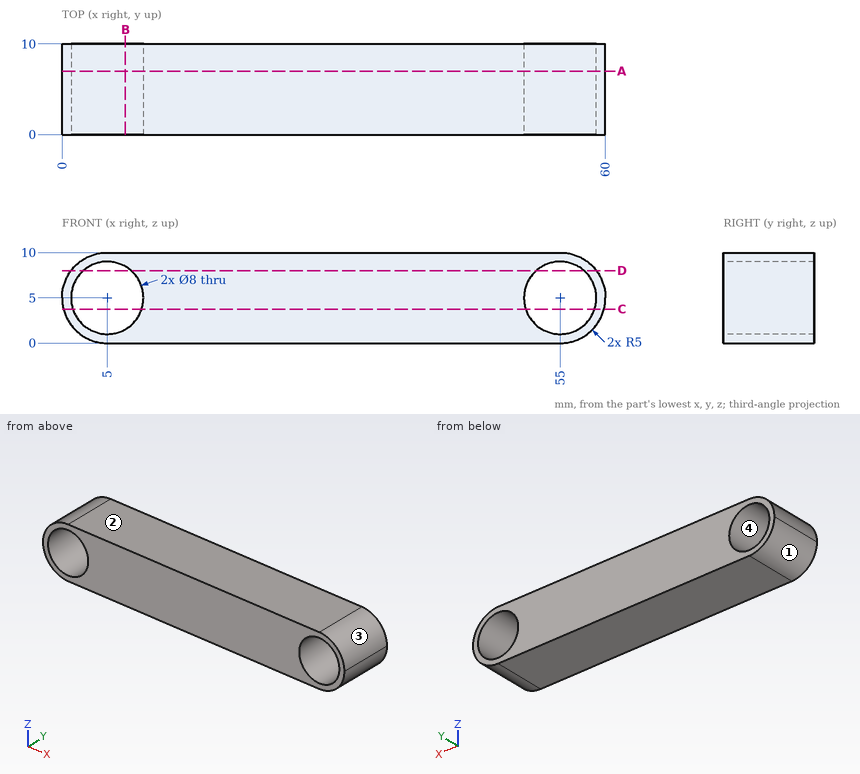
Here's the drawing with two shaded views (mm, measured from the low corner). I have some questions. Coordinates: 2 decimals unless noted, no trailing zeros. Write each loop counter-clockwise with the first axis right and the second up, starting at its lowest first coordinate (ties: lowest second). Pieces come first, ordered by that corner, then holes.
Item 1: I want a section at D-D on z = 8. Write out the boundary of the cut face in (x, y).
Item 2: I want a section at B-B on x = 7. Write out the boundary of the cut face in (y, z).
Item 3: I want a section at A-A on y = 7. Count the separate pieces of the cut face and the enclosed holes in it, and give its area (3 significant figures).
Item 4: I want a section at C-C on z = 3.75. Write out the boundary of the cut face in (x, y).
Item 5: If I drill on line 1 (X direction, y = 1.5, z = 4.75); line 2 (Z direction, x = 5, y = 8); line 3 (X direction, y = 9.25, z = 2), over which ranges is the centre line in solid material (lowest first)?
Item 6: If we mould it in two halves opening along X, with no side actions, what happens to the marked faces 1, 2, 3 and 4? For each: +X half, -X half, draft (parallel to the pull), parting line (faces both ways), or undercut.
Item 7: Will this pin go through, and if not, where does the flat tip stop? pin 1 (1.5 mm diameter, centred on y = 2, z = 3.5, fed in from +X).
Findings below:
1. outline: (1, 0) - (2.35, 0) - (2.35, 10) - (1, 10) - close; (7.65, 0) - (52.35, 0) - (52.35, 10) - (7.65, 10) - close; (57.65, 0) - (59, 0) - (59, 10) - (57.65, 10) - close
2. outline: (0, 0) - (10, 0) - (10, 1.54) - (0, 1.54) - close; (0, 8.46) - (10, 8.46) - (10, 10) - (0, 10) - close
3. separate pieces: 1
3. enclosed holes: 2
3. area: 478 mm2
4. outline: (0.16, 0) - (1.2, 0) - (1.2, 10) - (0.16, 10) - close; (8.8, 0) - (51.2, 0) - (51.2, 10) - (8.8, 10) - close; (58.8, 0) - (59.84, 0) - (59.84, 10) - (58.8, 10) - close
5. line 1: x = 0.01 to 1.01, 8.99 to 51.01, 58.99 to 59.99
5. line 2: z = 0 to 1, 9 to 10
5. line 3: x = 1 to 2.35, 7.65 to 52.35, 57.65 to 59
6. face 1: -X half
6. face 2: draft
6. face 3: +X half
6. face 4: undercut
7. pin 1: stops at x = 59.94
